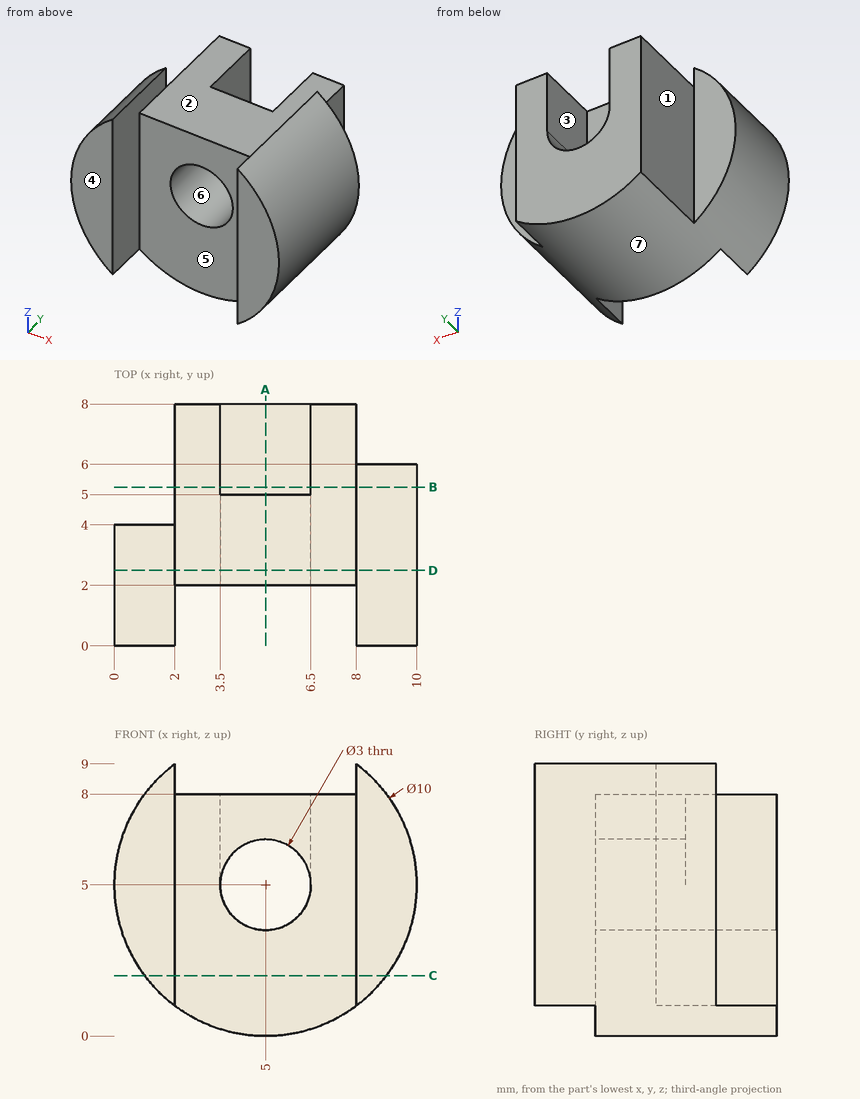
Part print with two shaded views. Sizes in mm from the minimum x, y, z corner. A direction names the side the tool comes from. Coordinates: 2 decimals unless noted, no trailing zeros. Order: outer loops, then holes, each group sorted by start corner. A loop starts at its lowest first (then second) coordinate and runs counter-clockwise, first axis right, second up. Notation, with made-up numbers: (68.25, 69) - (110.25, 69) arc R32 ccw to (110.25, 96) - close; hole circle Ø7 at (-30, 77). An arc over 180 degrees is marked (long way). Write item = value, one per line. Start each with the question number.
1) 3-axis set-ups, long thin cutter, end or side, ignore diameter. For the marked faces 1, 2 and 3: which of +Z, -Z, +X, -X, +Y, -Y reach the whole face in a straight line?
2) Saw through at C-C on z = 2. Write the cut outline in (x, y).
3) Two-plate mould, pull along X, no slides. Class the marked faces 4, 5, 6 and 7: pulls with the +X half, pulls with the -X half, needs draft (parallel to the pull), parting line crosses it, or undercut.
4) Saw through at B-B on y = 5.25. Write the cut outline in (x, z), then the cut area to 3 significant figures.
5) Saw through at A-A on x = 5. Write the cut outline in (y, z).
6) Saw through at D-D on y = 2.5. Write the cut outline in (x, z).
7) Flat gauge pins, fed straight in: pin 1 Ø3 at (x, z) = (6, 2) entering from -Y; pin 2 Ø0.9 at (y, z) = (6, 6.5) entering from +X; pin 3 Ø4 at (y, z) = (4, 1.5) entering from -X; pin 4 Ø2.5 at (x, z) = (5, 5) entering from +Y. Where does each tip first touch, or does it go through?
8) Wall check: line 1 along X through (y, z) = (3.95, 5); line 2 along X through (y, z) = (4.15, 5); line 3 along Z through (x, y) = (5, 4.5). Give the ranges that are in metal, low to high. Write a range as from..to.
From the geometry:
q1.face_1 = +Z, -Z, -X, +Y
q1.face_2 = +Z, +Y, -Y
q1.face_3 = +Z, +Y
q2.outline = (1, 0) - (2, 0) - (2, 2) - (8, 2) - (8, 0) - (9, 0) - (9, 6) - (8, 6) - (8, 8) - (2, 8) - (2, 4) - (1, 4) - close
q3.face_4 = needs draft
q3.face_5 = undercut
q3.face_6 = undercut
q3.face_7 = parting line crosses it
q4.outline = (2, 1) arc R5 ccw to (8, 9) - (8, 8) - (6.5, 8) - (6.5, 5) arc R1.5 cw to (3.5, 5) - (3.5, 8) - (2, 8) - close
q4.area = 44.7 mm^2
q5.outline = (2, 0) - (8, 0) - (8, 3.5) - (2, 3.5) - close; (2, 6.5) - (5, 6.5) - (5, 8) - (2, 8) - close
q6.outline = (2, 8) - (2, 9) arc R5 ccw (long way) to (8, 9) - (8, 8) - close; hole circle Ø3 at (5, 5)
q7.pin_1 = 2
q7.pin_2 = 9.89
q7.pin_3 = 0.23
q7.pin_4 = through
q8.line_1 = 0..3.5, 6.5..10
q8.line_2 = 2..3.5, 6.5..10
q8.line_3 = 0..3.5, 6.5..8
